```python
from build123d import *
from build123d import SkipClean  # not in build123d's __all__

# Parameters (mm, degrees)
F0_R             = 275
F1_DEPTH         = 25
F3_D             = 17.5
F3_COPIES_COUNT  = 8
F4_R             = 225
F5_DEPTH         = 5
F6_R             = 215
F7_DEPTH         = 30.001
F8_R             = 235
F8_R_2           = 215
F9_DEPTH         = 80
F10_R            = 282.5
F10_R_2          = 235
F10_R_3          = 215
F11_DEPTH        = 25
F13_D            = 17.5
F13_DEPTH        = 25
F13_TIP          = 5.2575304165
F13_COPIES_COUNT = 16


# Not quite as in the source:
# - after a boolean that leaves OpenCascade's solid faulty, fix() repairs it
# - a pattern or mirror of a feature is missing from the dataset's text; its kind, count and spacing are read off the source's solid


with BuildPart() as f1:
    # F0 (on Front) → F1 (new body)
    with BuildSketch(Plane.XZ):
        Circle(F0_R)
    extrude(amount=F1_DEPTH)

    # F3 (through all)
    with Locations(Plane.XZ.offset(25)):
        with Locations((95.6708580913, 230.9698831278)):
            f3 = Hole(F3_D / 2)

    # F3_copies: F3 ×8 about axis
    f3_copies_axis = Axis((0, 0, 0), (0, 1, 0))
    for i in range(1, F3_COPIES_COUNT):
        add(f3.rotate(f3_copies_axis, i * 360 / F3_COPIES_COUNT), clean=False, mode=Mode.SUBTRACT)

    # F4 (on face) → F5 (join)
    with BuildSketch(Plane.XZ.offset(25)):
        Circle(F4_R)
    extrude(amount=F5_DEPTH)

    # F6 (on face) → F7 (cut, through all)
    with BuildSketch(Plane.XZ.offset(30)):
        Circle(F6_R)
    extrude(amount=-F7_DEPTH, mode=Mode.SUBTRACT)

    # F8 (on face) → F9 (join)
    with BuildSketch(Plane(origin=(0, 0, 0), x_dir=(-1, 0, 0), z_dir=(0, 1, 0))):
        Circle(F8_R)
        Circle(F8_R_2, mode=Mode.SUBTRACT)
    with SkipClean():  # cleaning this boolean's faces spoils the solid; the shape is the same uncleaned
        extrude(amount=F9_DEPTH)

    # F10 (on face) → F11 (join)
    with BuildSketch(Plane(origin=(0, 80, 0), x_dir=(-1, 0, 0), z_dir=(0, 1, 0))):
        Circle(F10_R)
        Circle(F10_R_2, mode=Mode.SUBTRACT)
        Circle(F10_R_2)
        Circle(F10_R_3, mode=Mode.SUBTRACT)
    extrude(amount=F11_DEPTH)

    add(f1.part.fix(), mode=Mode.REPLACE)

    # F13
    with Locations(Plane(origin=(0, 105, 0), x_dir=(-1, 0, 0), z_dir=(0, 1, 0))):
        with Locations((0, 257.5)):
            f13 = Hole(F13_D / 2, depth=F13_DEPTH)
            with Locations((0, 0, -(F13_DEPTH + F13_TIP / 2))):  # 118° drill point
                Cone(0, F13_D / 2, F13_TIP, mode=Mode.SUBTRACT)

    # F13_copies: F13 ×16 about axis
    f13_copies_axis = Axis((0, 0, 0), (0, 1, 0))
    for i in range(1, F13_COPIES_COUNT):
        add(f13.rotate(f13_copies_axis, i * 360 / F13_COPIES_COUNT), clean=False, mode=Mode.SUBTRACT)


solid = f1.part
```
Source: CAD feature listing. Evaluate the final solid. Frame: model axes, mm. A direction names the side the tool comes from. Round coordinates to 2 decimals unless told otherwise and drop trailing zeros. Loops run counter-clockwise (first coordinate to the right, second up) from the corner with the lowest first, then second, coordinate; pieces in that order, holes last. Notation, with made-up numbers: M -29,45 L 30,45 A18 ccw 30,49 Z; hole C 47,-26 d10. An arc over 180 degrees is marked long. Use a Markdown table: item, result. Add a question column.
1. Cut plane B-B, the plane x = 31. Output: boundary loops of the cut face in (y, z).
2. Cut plane C-C, the plane z = 257.5. Output: boundary loops of the cut face in (x, y), and give its area (3 significant figures).
3. Contact query for flat-ended pins moving along their axis: pin 1 (8 mm diameter, centred on y = 75, z = 120, fed in from -X); pin 2 (10.5 mm diameter, centred on x = -237.9, z = 98.54, fed in from -Y); pin 3 (14 mm diameter, centred on x = 230.97, z = 95.67, fed in from -Y). Output: stop coordinate, or through.
4. Cut plane A-A, the plane z = 0. Output: boundary loops of the cut face in (x, y), and give its area (3 significant figures).
5. Pull-direction query (X, two-part tool) for faces 3 (the flat face through (-208, 105, -61)), 4 (the cylindrical face through (-224.782, -27.465, 9.893)), 5 (the cylindrical face through (239.645, -12.325, -96.81)); classes: +X half, -X half, draft (parallel to the pull), parting line (faces both ways), or undercut.
6. Ray query, line 1 along Y through (x, z) = (-86.5, -246); line 2 along Z through (x, y) = (101, -8); line 3 along X through (y, z) = (80.5, 230). Return the intervals inside material, ascending. Write a range as [from, to].
7. Cut plane D-D, the plane z = -164.5. Output: boundary loops of the cut face in (x, y), and give its area (3 significant figures).
8. Set-up query: faces 1 (the cylindrical face through (-89.76, -12.33, 237.42)), 2 (the cylindrical face through (-263.41, 92.32, -6.45)). Return all of +Z, -Z, +X, -X, +Y, -Y with unobstructed straight access to the full face (end or side cutting, diameter ignored); none if empty.
Solution:
| question | item | result |
|---|---|---|
| 1 | outline | M -30,-222.85 L -25,-222.85 L -25,-273.25 L 0,-273.25 L 0,-232.95 L 80,-232.95 L 80,-280.79 L 105,-280.79 L 105,-212.75 L -30,-212.75 Z; M -30,212.75 L 105,212.75 L 105,280.79 L 80,280.79 L 80,232.95 L 0,232.95 L 0,273.25 L -25,273.25 L -25,222.85 L -30,222.85 Z |
| 2 | outline | M -116.19,80 L -8.75,80 L -8.75,105 L -116.19,105 Z; M -96.53,-25 L 96.53,-25 L 96.53,0 L -96.53,0 Z; M 8.75,80 L 116.19,80 L 116.19,105 L 8.75,105 Z |
| 2 | area | 10,200 mm2 |
| 3 | pin 1 | stops at x = -204.37 |
| 3 | pin 2 | stops at y = -25 |
| 3 | pin 3 | stops at y = 80 |
| 4 | outline | M -282.5,80 L -266.25,80 L -266.25,105 L -282.5,105 Z; M -275,-25 L -225,-25 L -225,-30 L -215,-30 L -215,105 L -248.75,105 L -248.75,80 L -235,80 L -235,0 L -275,0 Z; M 215,-30 L 225,-30 L 225,-25 L 275,-25 L 275,0 L 235,0 L 235,80 L 248.75,80 L 248.75,105 L 215,105 Z; M 266.25,80 L 282.5,80 L 282.5,105 L 266.25,105 Z |
| 4 | area | 8,800 mm2 |
| 5 | face 3 | draft |
| 5 | face 4 | parting line |
| 5 | face 5 | undercut |
| 6 | line 1 | y = [-25, 0], [80, 105] |
| 6 | line 2 | z = [-255.78, -237.91], [-224.03, -189.8], [189.8, 224.03], [237.91, 255.78] |
| 6 | line 3 | x = [-164.03, -102.31], [-94.78, 94.78], [102.31, 164.03] |
| 7 | outline | M -229.66,80 L -167.82,80 L -167.82,0 L -220.37,0 L -220.37,-25 L -153.51,-25 L -153.51,-30 L -138.44,-30 L -138.44,105 L -229.66,105 Z; M 138.44,-30 L 153.51,-30 L 153.51,-25 L 220.37,-25 L 220.37,0 L 167.82,0 L 167.82,80 L 229.66,80 L 229.66,105 L 138.44,105 Z |
| 7 | area | 13,500 mm2 |
| 8 | face 1 | -Y |
| 8 | face 2 | +Y |
